from build123d import *

# Parameters (mm, degrees)
F0_R     = 3.175
F1_DEPTH = 25.4
F2_DEPTH = 25.4


with BuildPart() as f1:
    # F0 (on Front) → F1 (new body)
    with BuildSketch(Plane.XZ):
        with BuildLine():
            ThreePointArc((-9.4807107481, 63.7111065744), (-7.0521101036, 56.3910315801), (0, 53.2686379311))
            ThreePointArc((0, 53.2686379311), (6.7351920908, 56.0584458403), (9.525, 62.7936379311))
            ThreePointArc((9.525, 62.7936379311), (9.5142081889, 63.2469232041), (9.4818572097, 63.6991813339))
            ThreePointArc((9.4818572097, 63.6991813339), (0.0059901113, 72.3186360476), (-9.4807107481, 63.7111065744))
        make_face()
        with BuildLine():
            ThreePointArc((3.175, 62.7936379311), (2.2450640303, 60.5485739009), (0, 59.6186379311))
            ThreePointArc((0, 59.6186379311), (-2.2450640303, 65.0387019614), (3.175, 62.7936379311))
        make_face(mode=Mode.SUBTRACT)
        with BuildLine():
            ThreePointArc((9.525, 62.7936379311), (6.7351920908, 56.0584458403), (0, 53.2686379311))
            Line((0, 53.2686379311), (0, 27.8686379311))
            ThreePointArc((0, 27.8686379311), (7.8489973512, 25.7925098263), (13.6450153015, 20.1071564294))
            Line((13.6450153015, 20.1071564294), (9.4818572097, 63.6991813339))
            ThreePointArc((9.4818572097, 63.6991813339), (9.5142081889, 63.2469232041), (9.525, 62.7936379311))
        make_face()
        with BuildLine():
            Line((0, 27.8686379311), (0, 53.2686379311))
            ThreePointArc((0, 53.2686379311), (-7.0521101036, 56.3910315801), (-9.4807107481, 63.7111065744))
            Line((-9.4807107481, 63.7111065744), (-13.7112371906, 19.9947378369))
            ThreePointArc((-13.7112371906, 19.9947378369), (-7.9056360907, 25.7601386849), (0, 27.8686379311))
        make_face()
        with Locations((-5.4705687799, 41.0979501903)):
            Circle(F0_R, mode=Mode.SUBTRACT)
        with BuildLine():
            ThreePointArc((13.6450153015, 20.1071564294), (7.8489973512, 25.7925098263), (0, 27.8686379311))
            Line((0, 27.8686379311), (0, 15.1686379311))
            ThreePointArc((0, 15.1686379311), (2.2450640303, 14.2387019614), (3.175, 11.9936379311))
            ThreePointArc((3.175, 11.9936379311), (2.2450640303, 9.7485739009), (0, 8.8186379311))
            Line((0, 8.8186379311), (0, -3.8813620689))
            ThreePointArc((0, -3.8813620689), (10.1137339683, -0.2427018083), (15.5911917947, 9.005266565))
            ThreePointArc((15.5911917947, 9.005266565), (15.8038886787, 10.4927289966), (15.875, 11.9936379311))
            ThreePointArc((15.875, 11.9936379311), (15.3073551424, 16.2008345684), (13.6450153015, 20.1071564294))
        make_face()
        with BuildLine():
            Line((0, 15.1686379311), (0, 27.8686379311))
            ThreePointArc((0, 27.8686379311), (-7.9056360907, 25.7601386849), (-13.7112371906, 19.9947378369))
            ThreePointArc((-13.7112371906, 19.9947378369), (-15.5127721175, 15.3655107389), (-15.7954255641, 10.4061379311))
            ThreePointArc((-15.7954255641, 10.4061379311), (-10.6492737428, 0.2204228329), (0, -3.8813620689))
            Line((0, -3.8813620689), (0, 8.8186379311))
            ThreePointArc((0, 8.8186379311), (-3.175, 11.9936379311), (0, 15.1686379311))
        make_face()
        with BuildLine():
            ThreePointArc((0, -3.8813620689), (-10.6492737428, 0.2204228329), (-15.7954255641, 10.4061379311))
            Line((-15.7954255641, 10.4061379311), (-9.4772553384, -52.4588620689))
            ThreePointArc((-9.4772553384, -52.4588620689), (-7.063929059, -45.1167978232), (0, -41.9813620689))
            Line((0, -41.9813620689), (0, -3.8813620689))
        make_face()
        with BuildLine():
            ThreePointArc((15.5911917947, 9.005266565), (10.1137339683, -0.2427018083), (0, -3.8813620689))
            Line((0, -3.8813620689), (0, -41.9813620689))
            ThreePointArc((0, -41.9813620689), (6.7351920908, -44.7711699781), (9.525, -51.5063620689))
            Line((9.525, -51.5063620689), (36.5125, -51.5063620689))
            ThreePointArc((36.5125, -51.5063620689), (38.9380895153, -45.7947292849), (44.7324052746, -43.5738874543))
            Line((44.7324052746, -43.5738874543), (15.0507731119, -42.5171870062))
            ThreePointArc((15.0507731119, -42.5171870062), (9.1165249373, -39.5271472478), (7.5255613841, -33.075444052))
            Line((7.5255613841, -33.075444052), (15.5911917947, 9.005266565))
        make_face()
        with BuildLine():
            ThreePointArc((0, -41.9813620689), (-7.063929059, -45.1167978232), (-9.4772553384, -52.4588620689))
            ThreePointArc((-9.4772553384, -52.4588620689), (-6.3895642457, -58.5702911278), (0, -61.0313620689))
            Line((0, -61.0313620689), (0.6773435479, -61.0072478548))
            ThreePointArc((0.6773435479, -61.0072478548), (6.9705567315, -57.9976611571), (9.525, -51.5063620689))
            Line((9.525, -51.5063620689), (3.175, -51.5063620689))
            ThreePointArc((3.175, -51.5063620689), (-2.2450640303, -53.7514260991), (0, -48.3313620689))
            Line((0, -48.3313620689), (0, -41.9813620689))
        make_face()
        with BuildLine():
            Line((0.6773435479, -61.0072478548), (0, -61.0313620689))
            ThreePointArc((0, -61.0313620689), (0.3388863295, -61.0253316064), (0.6773435479, -61.0072478548))
        make_face()
        with BuildLine():
            Line((36.5125, -51.5063620689), (9.525, -51.5063620689))
            ThreePointArc((9.525, -51.5063620689), (6.9705567315, -57.9976611571), (0.6773435479, -61.0072478548))
            Line((0.6773435479, -61.0072478548), (26.128586054, -60.1011541732))
            Line((26.128586054, -60.1011541732), (44.7324052746, -59.4388366834))
            ThreePointArc((44.7324052746, -59.4388366834), (38.9380895153, -57.2179948528), (36.5125, -51.5063620689))
        make_face()
        with BuildLine():
            ThreePointArc((44.7324052746, -43.5738874543), (38.9380895153, -45.7947292849), (36.5125, -51.5063620689))
            ThreePointArc((36.5125, -51.5063620689), (38.9380895153, -57.2179948528), (44.7324052746, -59.4388366834))
            ThreePointArc((44.7324052746, -59.4388366834), (50.1616327839, -57.0182725536), (52.3875, -51.5063620689))
            ThreePointArc((52.3875, -51.5063620689), (50.1616327839, -45.9944515841), (44.7324052746, -43.5738874543))
        make_face()
        with BuildLine():
            ThreePointArc((47.625, -51.5063620689), (44.45, -54.6813620689), (41.275, -51.5063620689))
            ThreePointArc((41.275, -51.5063620689), (44.45, -48.3313620689), (47.625, -51.5063620689))
        make_face(mode=Mode.SUBTRACT)
    extrude(amount=F1_DEPTH)

    # F0 (on Front) → F2 (join)
    with BuildSketch(Plane.XZ):
        with BuildLine():
            ThreePointArc((9.525, -51.5063620689), (6.7351920908, -44.7711699781), (0, -41.9813620689))
            Line((0, -41.9813620689), (0, -48.3313620689))
            ThreePointArc((0, -48.3313620689), (2.2450640303, -49.2612980386), (3.175, -51.5063620689))
            Line((3.175, -51.5063620689), (9.525, -51.5063620689))
        make_face()
    extrude(amount=F2_DEPTH)


solid = f1.part
Design review of the part built by this model. Coordinates are the model's own, in mm. Coordinates: 2 decimals unless noted, no trailing zeros. Order: outer loops, then holes, each group sorted by start corner. A loop starts at its lowest first (then second) coordinate and runs counter-clockwise, first axis right, second up. Notation, with made-up numbers: (11, 8.25) -> (28, 8.25) arc R28 ccw to (28, 38.25) -> close; hole circle Ø8 at (85.25, -5). An arc over 180 degrees is marked (long way). Use one line per item in the form item = value. Start each with the question number.
(1) Insertion check: pin 1 (12 mm diameter, centred on y = -7, z = -25, fed in from +X); pin 2 (12 mm diameter, centred on x = 18.5, y = -16, fed in from -Z); pin 3 (1.5 mm diameter, centred on y = -5.5, z = 59, fed in from +X); pin 4 (5.5 mm diameter, centred on x = 44.45, z = -51.51, fed in from -Y). Each pin has a flat end and moves straight along its axis. Give the tip position at first contact, or say it passes through.
(2) Add section C-C on x = 17.5. State the section outline as (y, z) points, plus the area to 3 significant figures.
(3) The part is to be moulded in two halves that separate along X. For faces 1 (the cylindrical face through (42.74, -12.52, -48.83)), 2 (the flat face through (11.5, -12.52, -12.33)), 3 (the flat face through (3, 0, 7)), say which applies: +X half, -X half, draft (parallel to the pull), parting line (faces both ways), or undercut.
(4) Add section A-A on y = -18. Give the number of separate pieces and of enclosed holes in the cut face, plus the area to 3 significant figures.
(5) For probe 1 along Z at (x, y) = (44.45, -9.75); probe 2 along Z at (x, y) = (-4, -20); probe 3 along X at (y, z) = (-20.75, 53), list the stretches that pass through material, from the lowest coordinate up.
(6) Add section B-B on z = -15.5. State the section outline as (x, y) points, plus the area to 3 significant figures.
Answer block:
q1.pin_1 = 10.22
q1.pin_2 = -60.59
q1.pin_3 = 10
q1.pin_4 = through
q2.outline = (-25.4, -60.41) -> (0, -60.41) -> (0, -42.6) -> (-25.4, -42.6) -> close
q2.area = 452 mm²
q3.face_1 = undercut
q3.face_2 = +X half
q3.face_3 = draft
q4.separate_pieces = 1
q4.enclosed_holes = 5
q4.area = 3,590 mm²
q5.probe_1 = -59.45 to -54.68, -48.33 to -43.56
q5.probe_2 = -60.15 to 38.28, 43.91 to 71.44
q5.probe_3 = -10.52 to 10.5
q6.outline = (-13.19, -25.4) -> (10.89, -25.4) -> (10.89, 0) -> (-13.19, 0) -> close
q6.area = 612 mm²
